from build123d import *

# Parameters (mm, degrees)
F1_DEPTH = 10
F2_DEPTH = 25
F3_DEPTH = 25
F4_DEPTH = 25
F5_DEPTH = 25
F6_DEPTH = 25
F7_SIZE  = 5
F0_R     = 10
F8_DEPTH = 5


with BuildPart() as f1:
    # F0 (on Top) → F1 (new body)
    with BuildSketch(Plane.XY):
        Polygon((12.5, 38.4710442147), (-12.5, 38.4710442147), (-32.7254248594, 23.7764129074), (-40.4508497187, 0), (-32.7254248594, -23.7764129074), (-12.5, -38.4710442147), (12.5, -38.4710442147), (32.7254248594, -23.7764129074), (40.4508497187, 0), (32.7254248594, 23.7764129074), align=None)
        Polygon((-17.3205080757, 0), (-8.6602540378, 15), (8.6602540378, 15), (17.3205080757, 0), (8.6602540378, -15), (-8.6602540378, -15), align=None, mode=Mode.SUBTRACT)
    extrude(amount=F1_DEPTH)

    # F2 (add): a face of the model
    f2_faces = [f1.faces().sort_by_distance(p)[0] for p in [
        (36.5881372891, 11.8882064537, 5),
    ]]
    extrude(f2_faces, amount=F2_DEPTH)

    # F3 (add): a face of the model
    f3_faces = [f1.faces().sort_by_distance(p)[0] for p in [
        (0, 38.4710442147, 5),
    ]]
    extrude(f3_faces, amount=F3_DEPTH)

    # F4 (add): a face of the model
    f4_faces = [f1.faces().sort_by_distance(p)[0] for p in [
        (22.6127124297, -31.123728561, 5),
    ]]
    extrude(f4_faces, amount=F4_DEPTH)

    # F5 (add): a face of the model
    f5_faces = [f1.faces().sort_by_distance(p)[0] for p in [
        (-36.5881372891, 11.8882064537, 5),
    ]]
    extrude(f5_faces, amount=F5_DEPTH)

    # F6 (add): a face of the model
    f6_faces = [f1.faces().sort_by_distance(p)[0] for p in [
        (-22.6127124297, -31.123728561, 5),
    ]]
    extrude(f6_faces, amount=F6_DEPTH)

    # F7
    f7_edges = [f1.edges().sort_by_distance(p)[0] for p in [
        (-64.227263, 7.725425, 5),
        (-56.501838, 31.501838, 5),
        (-12.5, 63.471044, 5),
        (-47.420056, -44.001838, 5),
        (-27.194631, -58.696469, 5),
        (27.194631, -58.696469, 5),
        (64.227263, 7.725425, 5),
        (12.5, 63.471044, 5),
        (56.501838, 31.501838, 5),
        (47.420056, -44.001838, 5),
    ]]
    chamfer(f7_edges, length=F7_SIZE)

    # F0 (on Top) → F8 (join)
    with BuildSketch(Plane.XY):
        Polygon((8.6602540378, 15), (-8.6602540378, 15), (-17.3205080757, 0), (-8.6602540378, -15), (8.6602540378, -15), (17.3205080757, 0), align=None)
        Circle(F0_R, mode=Mode.SUBTRACT)
    extrude(amount=F8_DEPTH)


solid = f1.part
Could you check a few things on this model? Use its own coordinates, in mm. A direction names the side the tool comes from. Round coordinates to 2 decimals unless told otherwise and drop trailing zeros. Loops run counter-clockwise (first coordinate to the right, second up) from the corner with the lowest first, then second, coordinate; pieces in that order, holes last. Notation, with made-up numbers: (10, -24) - (37, -24) arc R12 ccw to (37, -7) - close; hole circle Ø3 at (74.5, -28). An arc over 180 degrees is marked (long way). Write item = value, one per line.
1) I'm going to push flat-ended pins straight in: P1, Ø1, axis at x = -6, z = 8, coming from the -Y side; P2, Ø5, axis at y = 47, z = 6, coming from the -X side; P3, Ø1, axis at y = 7, z = 7.5, coming from the +X side. Where does each tip first touch, or does it pass through?
Computed:
P1 = -38.47
P2 = -12.5
P3 = 60.14
2) On a 3-axis mill with a long thin cutter (end or side, diameter ignored), from which of +Z, -Z, +X, -X, +Y, -Y can I reach the whole of each face in a straight line? I mean faces 5 (the flat face through (-18.296, -46.448, 4.93)), 6 (the flat face through (-12.5, 48, 5)), 7 (the flat face through (36.534, -12.055, 4.93)). Say none if no direction works.
Computed:
face_5 = +Z, -Z, -Y
face_6 = +Z, -Z, -X, +Y
face_7 = +Z, -Z, +X
3) If we mould it in two halves opening along X, with no side actions, what happens to faces 1 (the flat face through (0, 15, 7)), 2 (the flat face through (-13.05, 7.4, 7.46)), 3 (the flat face through (38.52, -31.75, 4.93)), 4 (the flat face through (-49.828, 3.047, 4.93))? For each: pulls with the +X half, pulls with the -X half, needs draft (parallel to the pull), parting line crosses it, or undercut.
Computed:
face_1 = undercut
face_2 = undercut
face_3 = pulls with the +X half
face_4 = pulls with the -X half
4) Imagine slicing it at C-C (y = 4). Please give me the cut outline in (x, z).
Computed:
outline = (-52.76, 0) - (-9.17, 0) - (-9.17, 5) - (-15.01, 5) - (-15.01, 10) - (-52.76, 10) - close; (9.17, 0) - (52.76, 0) - (52.76, 10) - (15.01, 10) - (15.01, 5) - (9.17, 5) - close
5) Imagine slicing it at D-D (y = 43.5). Please give me the cut outline in (x, z).
Computed:
outline = (-12.5, 0) - (12.5, 0) - (12.5, 10) - (-12.5, 10) - close
6) I need wall thicknesses on line 1 along Y through (x, z) = (-1, 6.75); line 2 along Y through (x, z) = (0, 3.45); line 3 along X through (y, z) = (52.5, 5.75). Which ranges of each line are inside material? Lowest first, please. Write a range as from..to.
Computed:
line_1 = -38.47..-15, 15..63.47
line_2 = -38.47..-10, 10..63.47
line_3 = -12.5..12.5
7) Imagine slicing it at A-A (x = 0). Please give me the cut outline in (y, z).
Computed:
outline = (-38.47, 0) - (-10, 0) - (-10, 5) - (-15, 5) - (-15, 10) - (-38.47, 10) - close; (10, 0) - (63.47, 0) - (63.47, 10) - (15, 10) - (15, 5) - (10, 5) - close
